from build123d import *

# Parameters (mm, degrees)
SKETCH1_W           = 101.6
SKETCH1_H           = 59.6
BOSS_EXTRUDE1_DEPTH = 585.0001
SKETCH2_W           = 228.6
SKETCH2_H           = 21.5
CUT_EXTRUDE1_DEPTH  = 102.6
CUT_EXTRUDE4_DEPTH  = 6.35
CUT_EXTRUDE5_DEPTH  = 25.4
SKETCH6_R           = 4.934351916
CUT_EXTRUDE6_DEPTH  = 39.1


with BuildPart() as part:
    # Sketch1 → Boss-Extrude1 (new body)
    with BuildSketch(Plane.XY):
        with Locations((50.8, 29.8)):
            Rectangle(SKETCH1_W, SKETCH1_H)
    extrude(amount=BOSS_EXTRUDE1_DEPTH)

    # Sketch2 → Cut-Extrude1 (cut, through all)
    with BuildSketch(Plane.ZY):
        with Locations((304.8, 10.75)):
            Rectangle(SKETCH2_W, SKETCH2_H)
    extrude(amount=-CUT_EXTRUDE1_DEPTH, mode=Mode.SUBTRACT)

    # Sketch5 → Cut-Extrude4 (cut)
    with BuildSketch(Plane.ZY):
        with BuildLine():
            ThreePointArc((170, 31.35), (168.25, 29.6), (170, 27.85))
            ThreePointArc((170, 27.85), (171.75, 29.6), (170, 31.35))
        make_face()
        with BuildLine():
            ThreePointArc((110, 27.85), (111.75, 29.6), (110, 31.35))
            ThreePointArc((110, 31.35), (108.25, 29.6), (110, 27.85))
        make_face()
        with BuildLine():
            ThreePointArc((50, 27.85), (51.75, 29.6), (50, 31.35))
            ThreePointArc((50, 31.35), (48.25, 29.6), (50, 27.85))
        make_face()
        with BuildLine():
            ThreePointArc((530, 27.85), (531.75, 29.6), (530, 31.35))
            ThreePointArc((530, 31.35), (528.25, 29.6), (530, 27.85))
        make_face()
        with BuildLine():
            ThreePointArc((470, 27.85), (471.75, 29.6), (470, 31.35))
            ThreePointArc((470, 31.35), (468.25, 29.6), (470, 27.85))
        make_face()
        with BuildLine():
            ThreePointArc((410, 27.85), (411.75, 29.6), (410, 31.35))
            ThreePointArc((410, 31.35), (408.25, 29.6), (410, 27.85))
        make_face()
        with BuildLine():
            ThreePointArc((350, 27.85), (351.75, 29.6), (350, 31.35))
            ThreePointArc((350, 31.35), (348.25, 29.6), (350, 27.85))
        make_face()
        with BuildLine():
            ThreePointArc((290, 27.85), (291.75, 29.6), (290, 31.35))
            ThreePointArc((290, 31.35), (288.25, 29.6), (290, 27.85))
        make_face()
        with BuildLine():
            ThreePointArc((230, 27.85), (231.75, 29.6), (230, 31.35))
            ThreePointArc((230, 31.35), (228.25, 29.6), (230, 27.85))
        make_face()
    extrude(amount=-CUT_EXTRUDE4_DEPTH, mode=Mode.SUBTRACT)

    # Sketch5<3> → Cut-Extrude5 (cut)
    with BuildSketch(Plane.ZY):
        with BuildLine():
            ThreePointArc((562.7, 6.6), (566, 3.3), (569.3, 6.6))
            ThreePointArc((569.3, 6.6), (566, 9.9), (562.7, 6.6))
        make_face()
        with BuildLine():
            ThreePointArc((582.3, 6.6), (579, 9.9), (575.7, 6.6))
            ThreePointArc((575.7, 6.6), (579, 3.3), (582.3, 6.6))
        make_face()
        with BuildLine():
            ThreePointArc((575.7, 52.6), (579, 49.3), (582.3, 52.6))
            ThreePointArc((582.3, 52.6), (579, 55.9), (575.7, 52.6))
        make_face()
        with BuildLine():
            ThreePointArc((562.7, 52.6), (566, 49.3), (569.3, 52.6))
            ThreePointArc((569.3, 52.6), (566, 55.9), (562.7, 52.6))
        make_face()
        with BuildLine():
            ThreePointArc((6.7, 6.6), (10, 3.3), (13.3, 6.6))
            ThreePointArc((13.3, 6.6), (10, 9.9), (6.7, 6.6))
        make_face()
        with BuildLine():
            ThreePointArc((6.7, 52.6), (10, 49.3), (13.3, 52.6))
            ThreePointArc((13.3, 52.6), (10, 55.9), (6.7, 52.6))
        make_face()
    extrude(amount=-CUT_EXTRUDE5_DEPTH, mode=Mode.SUBTRACT)

    # Sketch6 → Cut-Extrude6 (cut, through all)
    with BuildSketch(Plane.XZ.offset(-21.5)):
        with Locations((50.8, 342.9)):
            Circle(SKETCH6_R)
        with Locations((50.8, 241.3)):
            Circle(SKETCH6_R)
    extrude(amount=-CUT_EXTRUDE6_DEPTH, mode=Mode.SUBTRACT)


solid = part.part
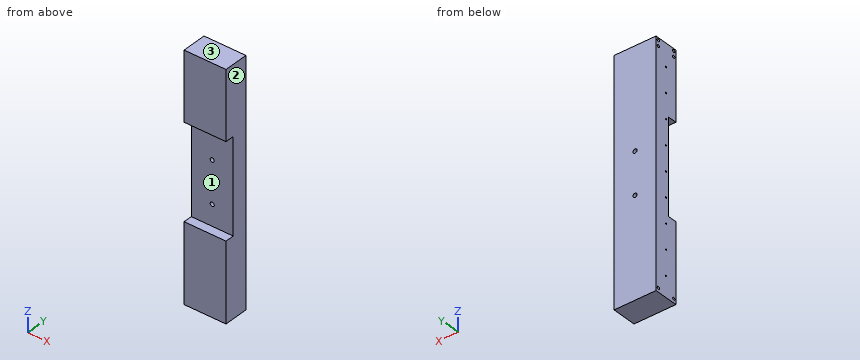
Geometry: final body of the model. Coordinates: model frame, mm. Face numbers are marked on the shaded views. Coordinates: 2 decimals unless noted, no trailing zeros. Order: outer loops, then holes, each group sorted by start corner. A loop starts at its lowest first (then second) coordinate and runs counter-clockwise, first axis right, second up.
(1) Section query A-A (x = 50.8). Return the cut outline in (y, z).
(2) Section query B-B (z = 342.9). Return the cut outline in (x, y), plus the area to 3 significant figures.
(3) Draft query along Z for the marked faces 1, 2 and 3. Return one class per face: pulls with the +Z half, pulls with the -Z half, needs draft (parallel to the pull), parting line crosses it, or undercut.
(4) Section query C-C (x = 78). Return the cut outline in (y, z).
(5) Material intervals for probe 1 along Z at (x, y) = (50.8, 46.5); probe 2 along Z at (x, y) = (7, 6) (3 decimals); probe 3 along Y at (x, z) = (17.75, 10), sorted ascending.
(6) First-contact query: pin 1 (6 mm diameter, centred on x = 15, z = 263.5, fed in from -Y); pin 2 (10.5 mm diameter, centred on y = 52.6, z = 579, fed in from -X); pin 3 (2 mm diameter, centred on y = 29.6, z = 290, fed in from -X). Flat tips, straight axial feed; report the tip coordinate or a pass-through.
Solution:
1. outline: (0, 0) - (59.6, 0) - (59.6, 236.37) - (21.5, 236.37) - (21.5, 190.5) - (0, 190.5) - close; (0, 419.1) - (21.5, 419.1) - (21.5, 347.83) - (59.6, 347.83) - (59.6, 585) - (0, 585) - close; (21.5, 246.23) - (59.6, 246.23) - (59.6, 337.97) - (21.5, 337.97) - close
2. outline: (0, 21.5) - (45.87, 21.5) - (45.87, 59.6) - (0, 59.6) - close; (55.73, 21.5) - (101.6, 21.5) - (101.6, 59.6) - (55.73, 59.6) - close
2. area: 3,490 mm2
3. face 1: undercut
3. face 2: needs draft
3. face 3: pulls with the +Z half
4. outline: (0, 0) - (59.6, 0) - (59.6, 585) - (0, 585) - (0, 419.1) - (21.5, 419.1) - (21.5, 190.5) - (0, 190.5) - close
5. probe 1: z = 0 to 236.37, 246.23 to 337.97, 347.83 to 585
5. probe 2: z = 0 to 6.755, 13.245 to 190.5, 419.1 to 562.755, 569.245 to 575.755, 582.245 to 585
5. probe 3: y = 0 to 3.3, 9.9 to 49.3, 55.9 to 59.6
6. pin 1: stops at y = 21.5
6. pin 2: stops at x = 0
6. pin 3: stops at x = 6.35
